```python
from build123d import *

# Parameters (mm, degrees)
SKETCH1_W           = 203.2
SKETCH1_H           = 101.6
SKETCH1_R           = 1.6
SKETCH1_W_2         = 68.58
SKETCH1_H_2         = 54.953705786
BOSS_EXTRUDE1_DEPTH = 3.175


with BuildPart() as part:
    # Sketch1 → Boss-Extrude1 (new body)
    with BuildSketch(Plane(origin=(0, 0, 0), x_dir=(1, 0, 0), z_dir=(0, 1, 0))):
        with Locations((101.6, -50.8)):
            Rectangle(SKETCH1_W, SKETCH1_H)
        with Locations(Location((20.431013284, -94.769213223, 0), (0, 0, 270))):
            Circle(SKETCH1_R, mode=Mode.SUBTRACT)
        with Locations(Location((20.431013284, -81.10763967, 0), (0, 0, 270))):
            Circle(SKETCH1_R, mode=Mode.SUBTRACT)
        with Locations(Location((85, -94.769213223, 0), (0, 0, 270))):
            Circle(SKETCH1_R, mode=Mode.SUBTRACT)
        with Locations(Location((85, -81.10763967, 0), (0, 0, 270))):
            Circle(SKETCH1_R, mode=Mode.SUBTRACT)
        with Locations(Location((96.6, -75.55, 0), (0, 0, 270))):
            Circle(SKETCH1_R, mode=Mode.SUBTRACT)
        Polygon((12.405089541, -78.276852893), (12.405089541, -74.276852893), (12.7, -74.276852893), (12.7, -27.323147107), (12.648382796, -27.323147107), (12.648382796, -23.323147107), (81.28, -23.323147107), (81.28, -78.276852893), align=None, mode=Mode.SUBTRACT)
        with Locations(Location((118.2, -94.769213223, 0), (0, 0, 270))):
            Circle(SKETCH1_R, mode=Mode.SUBTRACT)
        with Locations(Location((118.2, -81.10763967, 0), (0, 0, 270))):
            Circle(SKETCH1_R, mode=Mode.SUBTRACT)
        with Locations(Location((106.6, -75.55, 0), (0, 0, 270))):
            Circle(SKETCH1_R, mode=Mode.SUBTRACT)
        with Locations(Location((182.768986716, -94.769213223, 0), (0, 0, 270))):
            Circle(SKETCH1_R, mode=Mode.SUBTRACT)
        with Locations(Location((182.768986716, -81.10763967, 0), (0, 0, 270))):
            Circle(SKETCH1_R, mode=Mode.SUBTRACT)
        with Locations((156.21, -50.8)):
            Rectangle(SKETCH1_W_2, SKETCH1_H_2, mode=Mode.SUBTRACT)
        with Locations(Location((20.431013284, -20.49236033, 0), (0, 0, 270))):
            Circle(SKETCH1_R, mode=Mode.SUBTRACT)
        with Locations(Location((20.431013284, -6.830786777, 0), (0, 0, 270))):
            Circle(SKETCH1_R, mode=Mode.SUBTRACT)
        with Locations(Location((96.6, -26.05, 0), (0, 0, 270))):
            Circle(SKETCH1_R, mode=Mode.SUBTRACT)
        with Locations(Location((85, -20.49236033, 0), (0, 0, 270))):
            Circle(SKETCH1_R, mode=Mode.SUBTRACT)
        with Locations(Location((85, -6.830786777, 0), (0, 0, 270))):
            Circle(SKETCH1_R, mode=Mode.SUBTRACT)
        with Locations(Location((106.6, -26.05, 0), (0, 0, 270))):
            Circle(SKETCH1_R, mode=Mode.SUBTRACT)
        with Locations(Location((118.2, -20.49236033, 0), (0, 0, 270))):
            Circle(SKETCH1_R, mode=Mode.SUBTRACT)
        with Locations(Location((118.2, -6.830786777, 0), (0, 0, 270))):
            Circle(SKETCH1_R, mode=Mode.SUBTRACT)
        with Locations(Location((182.768986716, -20.49236033, 0), (0, 0, 270))):
            Circle(SKETCH1_R, mode=Mode.SUBTRACT)
        with Locations(Location((182.768986716, -6.830786777, 0), (0, 0, 270))):
            Circle(SKETCH1_R, mode=Mode.SUBTRACT)
    extrude(amount=-BOSS_EXTRUDE1_DEPTH)


solid = part.part
```
Build history of the part. All positions in model axes, mm. Round coordinates to 2 decimals unless told otherwise and drop trailing zeros. Loops run counter-clockwise (first coordinate to the right, second up) from the corner with the lowest first, then second, coordinate; pieces in that order, holes last.
Item 1: Drill centre lines: line 1 along X through (y, z) = (-2.2, 58); line 2 along X through (y, z) = (-1.6, 75.55); line 3 along Z through (x, y) = (50.5, -0.2). Where is each one in solid material? Low to high.
Item 2: Saw through at B-B (y = -1.6). State how many separate pieces and enclosed holes the cut face has, then the cut area to 3 significant figures.
Item 3: Saw through at A-A (x = 76). List the corners of the cut face in (y, z) (3 decimals), then the cut area to 3 significant figures.
Worked answers:
1. line 1: x = 0 to 12.7, 81.28 to 121.92, 190.5 to 203.2
1. line 2: x = 0 to 12.41, 81.28 to 95, 98.2 to 105, 108.2 to 121.92, 190.5 to 203.2
1. line 3: z = 0 to 23.32, 78.28 to 101.6
2. separate pieces: 1
2. enclosed holes: 22
2. area: 12,900 mm2
3. outline: (-3.175, 0) - (0, 0) - (0, 23.323) - (-3.175, 23.323) - close; (-3.175, 78.277) - (0, 78.277) - (0, 101.6) - (-3.175, 101.6) - close
3. area: 148 mm2
